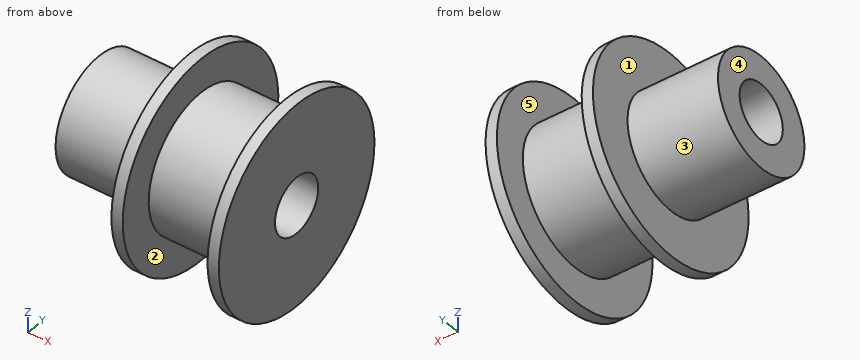
from build123d import *

# Parameters (mm, degrees)
F2_R     = 2.5
F3_DEPTH = 17.501


with BuildPart() as f1:
    # F0 (on Front) → F1 (revolve)
    with BuildSketch(Plane.XZ):
        Polygon((0, 5), (0, 0), (17.5, 0), (17.5, 9), (16.5, 9), (16.5, 6), (9, 6), (9, 9), (8, 9), (8, 5), align=None)
    revolve(axis=Axis((-7.792865, 0, 0), (-1, 0, 0)))

    # F2 (on face) → F3 (cut, through all)
    with BuildSketch(Plane(origin=(0, 0, 0), x_dir=(0, -1, 0), z_dir=(-1, 0, 0))):
        Circle(F2_R)
    extrude(amount=-F3_DEPTH, mode=Mode.SUBTRACT)


solid = f1.part
CAD build for the part. Positions are in the model's coordinates, mm. Face numbers are marked on the shaded views. A direction names the side the tool comes from. Give positions to 0.01 mm unless a question says otherwise; leave off trailing zeros. Loops run counter-clockwise (first coordinate to the right, second up) from the corner with the lowest first, then second, coordinate; pieces in that order, holes last. Notation, with made-up numbers: M 65.5,-9 L 84.5,-9 A28 cw 84.5,23 Z; hole C 13.5,14 d6. An arc over 180 degrees is marked long. Answer in a Markdown table with one row per item. Add a question column.
Item 1: Probe probe 1 along X at (y, z) = (1.75, -6.25); probe 2 along Z at (x, y) = (15.75, 1); probe 3 along Y at (x, z) = (6, 2.25). List the from-to ranges inside material, lowest first.
Item 2: Mould opens along X. For the marked faces 1, 2 and 3 say: +X half, -X half, draft (parallel to the pull), parting line (faces both ways), or undercut.
Item 3: Drop flat-ended pins along their axis: P1, Ø6, axis at x = 14, z = 6, coming from the +Y side; P2, Ø8, axis at x = 6, z = 4, coming from the +Y side. Give the stop position or say it passes through.
Item 4: Tool access for the marked faces 4 and 5: list every direction of +Z, -Z, +X, -X, +Y, -Y with a clear straight run to the whole face (end or side of a thin tool).
Item 5: Band-saw the part on A-A on z = 0. Give the cut face in (x, y), then the cut area to 4 significant figures.
Item 6: Band-saw the part on C-C on x = 1.75. Give the cut face in (y, z).
Item 7: Band-saw the part on D-D on z = 3.75. Give the cut face in (x, y).
Reply:
| question | item | result |
|---|---|---|
| 1 | probe 1 | x = 8 to 9, 16.5 to 17.5 |
| 1 | probe 2 | z = -5.92 to -2.29, 2.29 to 5.92 |
| 1 | probe 3 | y = -4.47 to -1.09, 1.09 to 4.47 |
| 2 | face 1 | -X half |
| 2 | face 2 | undercut |
| 2 | face 3 | draft |
| 3 | P1 | stops at y = 7.88 |
| 3 | P2 | stops at y = 8.98 |
| 4 | face 4 | +Z, -Z, -X, +Y, -Y |
| 4 | face 5 | none |
| 5 | outline | M 0,-5 L 8,-5 L 8,-9 L 9,-9 L 9,-6 L 16.5,-6 L 16.5,-9 L 17.5,-9 L 17.5,-2.5 L 0,-2.5 Z; M 0,2.5 L 17.5,2.5 L 17.5,9 L 16.5,9 L 16.5,6 L 9,6 L 9,9 L 8,9 L 8,5 L 0,5 Z |
| 5 | area | 118.5 mm^2 |
| 6 | outline | C 0,0 d10; hole C 0,0 d5 |
| 7 | outline | M 0,-3.31 L 8,-3.31 L 8,-8.18 L 9,-8.18 L 9,-4.68 L 16.5,-4.68 L 16.5,-8.18 L 17.5,-8.18 L 17.5,8.18 L 16.5,8.18 L 16.5,4.68 L 9,4.68 L 9,8.18 L 8,8.18 L 8,3.31 L 0,3.31 Z |
